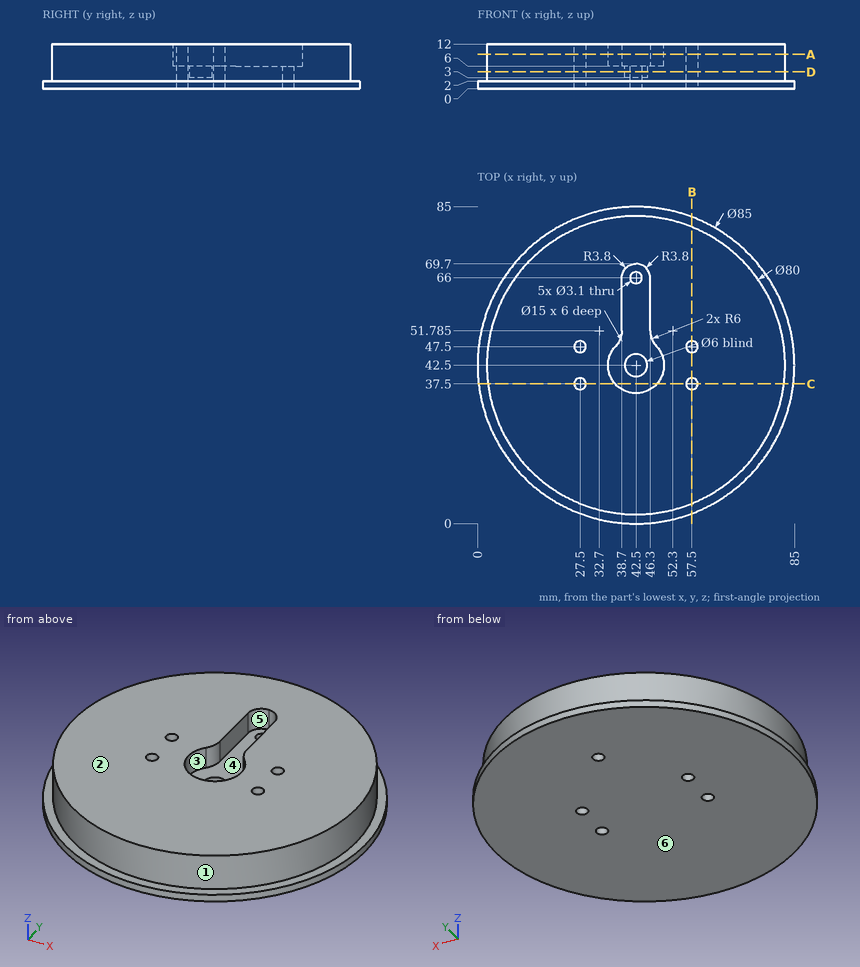
Verification items for this drawing (mm, ordinates from the low corner). A direction names the side the tool comes from. Give positions to 0.01 mm unless a question says otherwise; leave off trailing zeros. Write each loop counter-clockwise with the first axis right and the second up, starting at its lowest first coordinate (ties: lowest second). Pieces come first, ordered by that corner, then holes. Notation, with made-up numbers: (-32.75, 17) -> (22.25, 17) arc R24 ccw to (22.25, 55) -> close; hole circle Ø8 at (66.25, 66.25). An arc over 180 degrees is marked (long way). Use one line per item in the form item = value.
Item 1: Mould release check, pull along X, two halves, no side actions. Record for the marked faces 1, 2, 3 and 4: released by +X, released by -X, zero draft, split by the parting line, or undercut.
Results list:
face_1 = split by the parting line
face_2 = zero draft
face_3 = undercut
face_4 = undercut
Item 2: Sectioned sample at B-B on x = 57.5. Enter the section's corners in (y, z) (3 decimals).
Results list:
outline = (2.735, 0) -> (35.95, 0) -> (35.95, 12) -> (5.419, 12) -> (5.419, 2) -> (2.735, 2) -> close; (39.05, 0) -> (45.95, 0) -> (45.95, 12) -> (39.05, 12) -> close; (49.05, 0) -> (82.265, 0) -> (82.265, 2) -> (79.581, 2) -> (79.581, 12) -> (49.05, 12) -> close
Item 3: Scan lines: line 1 (Y direction, x = 42.5, z = 4.3); line 2 (Y direction, x = 42.5, z = 1.9); line 3 (Y direction, x = 42.5, z = 2.8). Record each from-to range of solid material in increasing order.
Results list:
line_1 = 2.5 to 39.5, 45.5 to 64.45, 67.55 to 82.5
line_2 = 0 to 64.45, 67.55 to 85
line_3 = 2.5 to 64.45, 67.55 to 82.5
Item 4: Sectioned sample at C-C on y = 37.5. Enter the section's corners in (x, z) (3 decimals), plus the area to 3 significant figures.
Results list:
outline = (0.295, 0) -> (25.95, 0) -> (25.95, 12) -> (2.814, 12) -> (2.814, 2) -> (0.295, 2) -> close; (29.05, 0) -> (55.95, 0) -> (55.95, 12) -> (48.09, 12) -> (48.09, 6) -> (36.91, 6) -> (36.91, 12) -> (29.05, 12) -> close; (59.05, 0) -> (84.705, 0) -> (84.705, 2) -> (82.186, 2) -> (82.186, 12) -> (59.05, 12) -> close
area = 821 mm2
Item 5: Sectioned sample at A-A on z = 9.25. Count the separate pieces of the cut face and the enclosed holes in it, plus the area to 3 significant figures.
Results list:
separate_pieces = 1
enclosed_holes = 5
area = 4,670 mm2
Item 6: Sectioned sample at D-D on z = 4.5. Enter the section's corners in (x, y).
Results list:
outline = circle Ø80 at (42.5, 42.5); hole circle Ø3.1 at (27.5, 37.5); hole circle Ø3.1 at (27.5, 47.5); hole circle Ø6 at (42.5, 42.5); hole circle Ø3.1 at (42.5, 66); hole circle Ø3.1 at (57.5, 37.5); hole circle Ø3.1 at (57.5, 47.5)
Item 7: Access from +Z, -Z, +X, -X, +Y, -Y to the whole of each face (thin tool, end or side, straight path). Record for the marked faces 5 and 6.
Results list:
face_5 = +Z
face_6 = -Z, +X, -X, +Y, -Y
Item 8: Depth check by flat-ended pin: pin 1 Ø6.5 at (y, z) = (62, 9) entering from -X; pin 2 Ø3 at (x, y) = (44, 43) entering from +Z; pin 3 Ø5.5 at (x, y) = (42.5, 42.5) entering from +Z. Enter the tip coordinate at first touch or a pass-through.
Results list:
pin_1 = 5.95
pin_2 = 6
pin_3 = 3
